Autodesk Inventor part; units mm, degrees
ref_plane "YZ Plane" through (0, 0, 0) normal (1, 0, 0) x (0, 1, 0)
ref_plane "XZ Plane" through (0, 0, 0) normal (0, 1, 0) x (-1, 0, 0)
ref_plane "XY Plane" through (0, 0, 0) normal (0, 0, 1) x (1, 0, 0)
sketch "Sketch1" plane through (0, 0, 0) normal (0, 0, 1) x (1, 0, 0)
  line L0 (60, -5.875) -> (-60, -5.875)
  line L1 (-60, -5.875) -> (-60, 5.875)
  line L2 (-60, 5.875) -> (60, 5.875)
  line L3 (60, 5.875) -> (60, -5.875)
  line L4 (60, -5.875) -> (-60, 5.875) construction
  line L5 (-60, -5.875) -> (60, 5.875) construction
  point P0 (0, 0)
  dimension "d0" = 120
  dimension "d1" = 11.75
extrude "Extrusion1" add sketch "Sketch1" along normal blind 25
fillet "Fillet1" radius 8 2 edges at (60, 0, 25) (-60, 0, 25)
chamfer "Chamfer1" distance 2 angle 45 5 edges at (60, -5.875, 8.5) (57.6569, -5.875, 22.6569) (0, -5.875, 25) (-57.6569, -5.875, 22.6569) (-60, -5.875, 8.5)
sketch "Sketch2" plane through (0, 0, 25) normal (0, 0, 1) x (1, 0, 0)
  line L0 (-53, 0.125) -> (-37, 0.125) construction
  line L1 (-52, -5.875) -> (52, -5.875)
  line L2 (-60, 5.875) -> (-60, -3.875)
  line L3 (37, 0.125) -> (53, 0.125) construction
  line L4 (60, -3.875) -> (60, 5.875)
  point P0 (-45, 0.125)
  point P1 (45, 0.125)
  dimension "d8" = 16
  dimension "d9" = 6
  dimension "d35" = 15
  dimension "d36" = 15
  dimension "d37" = 90
hole "Hole1" at (-53, 0.125, 25) at (-37, 0.125, 25) at (37, 0.125, 25) at (53, 0.125, 25) direction (0, 0, -1) diameter 5.3 end through all counterbore diameter 9 counterbore depth 5
sketch "Sketch3" plane through (-60, 5.875, 0) normal (0, 1, 0) x (1, 0, 0)
  point P0 (60, 0)
  point P1 (105, -15)
  point P2 (15, -15)
  point P3 (15, -25)
  point P4 (105, -25)
  dimension "d22" = 10
hole "Hole2" at (45, 5.875, 15) at (-45, 5.875, 15) direction (0, -1, 0) diameter 5.3 end through all
sketch "Sketch4" plane through (-58, -5.875, 0) normal (0, -1, 0) x (1, 0, 0)
  circle A0 centre (13, 15) radius 2.65
  circle A1 centre (103, 15) radius 2.65
  line L0 (0, 0) -> (0, 17)
  line L1 (0, 0) -> (116, 0)
  line L2 (116, 17) -> (116, 0)
  arc A2 (116, 17) -> (110, 23) centre (110, 17) ccw
  line L3 (6, 23) -> (110, 23)
  arc A3 (6, 23) -> (0, 17) centre (6, 17) ccw
  line L4 (107.125, 12.6184) -> (103, 10.2369)
  line L5 (103, 10.2369) -> (98.875, 12.6184)
  line L6 (98.875, 12.6184) -> (98.875, 17.3816)
  line L7 (98.875, 17.3816) -> (103, 19.7631)
  line L8 (103, 19.7631) -> (107.125, 17.3816)
  line L9 (107.125, 17.3816) -> (107.125, 12.6184)
  line L10 (8.875, 17.3816) -> (13, 19.7631)
  line L11 (13, 19.7631) -> (17.125, 17.3816)
  line L12 (17.125, 17.3816) -> (17.125, 12.6184)
  line L13 (17.125, 12.6184) -> (13, 10.2369)
  line L14 (13, 10.2369) -> (8.875, 12.6184)
  line L15 (8.875, 12.6184) -> (8.875, 17.3816)
  point P0 (58, 0)
  dimension "d30" = 8.25
extrude "Extrusion2" cut sketch "Sketch4" against normal blind 5 contours A0 | A1 | L4 L5 L6 L7 L8 L9 | L10 L11 L12 L13 L14 L15
properties part number "Door Bar Brace Mount" material "ABS Plastic"
Geometry: final body of the model. Coordinates: model frame, mm. A direction names the side the tool comes from. Give positions to 0.01 mm unless a question says otherwise; leave off trailing zeros. Loops run counter-clockwise (first coordinate to the right, second up) from the corner with the lowest first, then second, coordinate; pieces in that order, holes last. Notation, with made-up numbers: M 88,21 L 140,21 A23 cw 140,33 Z; hole C -7.75,-32 d11. An arc over 180 degrees is marked long. Put each result on its own line as item: value. Start each with the question number.
1) Access query for faces 1 (the flat face through (42.909, -3.41, 18.556)), 2 (the flat face through (-35, -2, 20)), 3 (the flat face through (-59.014, -4.861, 8.381)). Directions: +Z, -Z, +X, -X, +Y, -Y. A direction counts if a zero-diameter tool reaches every point of the face in a straight line with its end or side. Return the directions, or none.
2) Ray query, line 1 along X through (y, z) = (0, 11); line 2 along Y through (x, z) = (-53, 21.5) (3 decimals); line 3 along X through (y, z) = (-2, 4.75). Return the intervals inside material, ascending.
3) Contact query for flat-ended pins moving along their axis: pin 1 (7 mm diameter, centred on x = -37, y = 0.125, fed in from +Z); pin 2 (2.5 mm diameter, centred on x = -46, z = 16.5, fed in from -Y) (3 decimals); pin 3 (5 mm diameter, centred on y = 1, z = 20.5, fed in from +X). Output: stop coordinate, or through.
4) Pull-direction query (X, two-part tool) for faces 4 (the cylindrical face through (-58.6, 1.07, 21.52)), 5 (the cylindrical face through (-55.627, 0.47, 9.86)), 6 (the flat face through (1, -5.875, 11)), 7 (the flat face through (60, 1, 8)); classes: pulls with the +X half, pulls with the -X half, needs draft (parallel to the pull), parting line crosses it, or undercut.
5) Cut plane D-D (y = 1.25). Give the number of separate pieces and of enclosed holes in the cut face, then the cut area to 3 significant figures.
6) Cut plane A-A (z = 15). Output: boundary loops of the cut face in (x, y) (3 decimals).
7) Cut plane C-C (z = 4.75). Output: boundary loops of the cut face in (x, y) (3 decimals).
8) Cut plane B-B (x = -37). Output: boundary loops of the cut face in (y, z) (3 decimals), then the cut area to 3 significant figures.
Verdict:
1. face 1: -Y
1. face 2: +Z
1. face 3: +Z, -Z, -X, -Y
2. line 1: -60 to -55.65, -50.35 to -39.65, -34.35 to 34.35, 39.65 to 50.35, 55.65 to 60
2. line 2: -5.875 to -4.375, 4.625 to 5.875
2. line 3: -60 to -54.58, -51.42 to -38.58, -35.42 to 35.42, 38.58 to 51.42, 54.58 to 60
3. pin 1: z = 20
3. pin 2: y = -0.875
3. pin 3: x = 59.94
4. face 4: pulls with the -X half
4. face 5: undercut
4. face 6: needs draft
4. face 7: pulls with the +X half
5. separate pieces: 5
5. enclosed holes: 2
5. area: 2,380 mm2
6. outline: M -60,-3.875 L -58,-5.875 L -49.125,-5.875 L -49.125,-0.875 L -47.65,-0.875 L -47.65,5.875 L -60,5.875 Z; M -42.35,-0.875 L -40.875,-0.875 L -40.875,-5.875 L 40.875,-5.875 L 40.875,-0.875 L 42.35,-0.875 L 42.35,5.875 L -42.35,5.875 Z; M 47.65,-0.875 L 49.125,-0.875 L 49.125,-5.875 L 58,-5.875 L 60,-3.875 L 60,5.875 L 47.65,5.875 Z; hole C -53,0.125 d5.3; hole C -37,0.125 d5.3; hole C 37,0.125 d5.3; hole C 53,0.125 d5.3
7. outline: M -60,-3.875 L -58,-5.875 L 58,-5.875 L 60,-3.875 L 60,5.875 L -60,5.875 Z; hole C -53,0.125 d5.3; hole C -37,0.125 d5.3; hole C 37,0.125 d5.3; hole C 53,0.125 d5.3
8. outline: M -5.875,0 L -2.525,0 L -2.525,20 L -4.375,20 L -4.375,24.5 L -5.875,23 Z; M 2.775,0 L 5.875,0 L 5.875,25 L 4.625,25 L 4.625,20 L 2.775,20 Z
8. area: 141 mm2
